The model under review builds one solid part; all positions refer to its coordinate system, in mm. A direction names the side the tool comes from. Round coordinates to 2 decimals unless told otherwise and drop trailing zeros. Order: outer loops, then holes, each group sorted by start corner. A loop starts at its lowest first (then second) coordinate and runs counter-clockwise, first axis right, second up. Notation, with made-up numbers: (-39.5, -10.5) - (9.5, -10.5) arc R16 ccw to (9.5, -4.5) - close; hole circle Ø5 at (87, 48.25). An arc over 180 degrees is marked (long way). One line per question, with ' | ' between items. Start each with the question number.
Item 1: Add section B-B on x = -27.5. State the section outline as (y, z) points.
Item 2: Insertion check: pin 1 Ø3.5 at (y, z) = (-35.5, -5) entering from -X; pin 2 Ø2.5 at (y, z) = (-34.5, -23) entering from +X; pin 3 Ø3.5 at (y, z) = (-35, -6.5) entering from +X. Each pin has a flat end and moves straight along its axis. Give the tip position at first contact, or say it passes through.
Item 3: Add section A-A on z = -4.5. State the section outline as (x, y) points.
Item 4: Draft analysis for pull direction Y (two halves, no side actions). For faces 4 (the face through (-30, 35, -1.58)), 5 (the face through (-16, 36.25, -12)), 6 (the face through (80, 0, -4)), state which applies: +Y half, -Y half, draft (parallel to the pull), parting line (faces both ways), or undercut.
Item 5: For L1, parallel to Y at x = -38, z = -30.5; L2, parallel to X at y = -28, z = -2; L3, parallel to X at y = -30, z = -9.5, list the stretches that pass through material, from the lowest coordinate up. Write a range as [from, to].
Item 6: Tool access review of faces 1 (the face through (-66, -35, -1.093)), 2 (the face through (-80, 0, -17)), 3 (the face through (-47.3, 35, -17)): name each direction out of +Z, -Z, +X, -X, +Y, -Y from which nothing blocks a thin tool from reaching the whole face with its end or side.
Item 7: Add section C-C on y = 6.5. State the section outline as (x, z) points, and give its area (3 significant figures).
Item 8: Add section D-D on x = -9. State the section outline as (y, z) points, and give its area (3 significant figures).
from build123d import *

# Parameters (mm, degrees)
ESQUISSE1_W                  = 160
ESQUISSE1_H                  = 66.5
BOSS_EXTRU_1_DEPTH           = 3
ESQUISSE3_W                  = 3
ESQUISSE3_H                  = 70.75
BOSS_EXTRU_2_DEPTH           = 33
ESQUISSE5_W                  = 166
ESQUISSE5_H                  = 33
ESQUISSE5_W_2                = 11.569169734
ESQUISSE5_H_2                = 9.894756015
BOSS_EXTRU_3_DEPTH           = 3
ENL_V_MAT_EXTRU_1_DEPTH      = 500
ENL_V_MAT_EXTRU_1_DEPTH_BACK = 13
ESQUISSE6_W                  = 33
ESQUISSE6_H                  = 1.25
CONG_2_R                     = 4
ESQUISSE7_W                  = 98.078954594
ESQUISSE7_H                  = 17.67
ENL_V_MAT_EXTRU_2_DEPTH      = 103
ESQUISSE8_R                  = 3.75
ENL_V_MAT_EXTRU_3_DEPTH      = 60
ESQUISSE9_W                  = 103.919717687
ESQUISSE9_H                  = 4.5
ENL_V_MAT_EXTRU_4_DEPTH      = 90
ESQUISSE11_W                 = 11.569169734
ESQUISSE11_H                 = 9.894756015
BOSS_EXTRU_4_DEPTH           = 3
D_PLACER_START               = -33.9
D_PLACER_LA_FACE2_DEPTH      = 3.9
ESQUISSE13_W                 = 16.502074088
ESQUISSE13_H                 = 4.3431
ENL_V_MAT_EXTRU_5_DEPTH      = 10
ESQUISSE15_W                 = 9.760998185
ESQUISSE15_H                 = 7
ENL_V_MAT_EXTRU_6_DEPTH      = 10


# Read off the part's stored shape, not the designer's step: Déplacer la face2
with BuildPart() as part:
    # Esquisse1 → Boss.-Extru.1 (new body)
    with BuildSketch(Plane.XY):
        Rectangle(ESQUISSE1_W, ESQUISSE1_H)
    extrude(amount=BOSS_EXTRU_1_DEPTH)

    # Esquisse3 → Boss.-Extru.2 (add)
    with BuildSketch(Plane.XY.offset(3)):
        with Locations((-81.5, -2.125)):
            Rectangle(ESQUISSE3_W, ESQUISSE3_H)
    boss_extru_2 = extrude(amount=-BOSS_EXTRU_2_DEPTH)

    # Symétrie1: Boss.-Extru.2 across plane
    add(boss_extru_2.mirror(Plane(origin=(0, 0, 0), x_dir=(0, 0, 1), z_dir=(1, 0, 0))))

    # Esquisse5 → Boss.-Extru.3 (add)
    with BuildSketch(Plane(origin=(0, 33.25, 0), x_dir=(1, 0, 0), z_dir=(0, 1, 0))):
        with Locations((0, 13.5)):
            Rectangle(ESQUISSE5_W, ESQUISSE5_H)
        with Locations((-29.852297111, 6.527378008)):
            Rectangle(ESQUISSE5_W_2, ESQUISSE5_H_2, mode=Mode.SUBTRACT)
    boss_extru_3 = extrude(amount=BOSS_EXTRU_3_DEPTH)

    # Symétrie2: Boss.-Extru.3 across plane
    add(boss_extru_3.mirror(Plane(origin=(0, 0, 0), x_dir=(0, 0, 1), z_dir=(0, -1, 0))))

    # Esquisse6 → Enlèv. mat.-Extru.1 (cut, two sides: drawn at the far end of the back side and taken through both)
    with BuildSketch(Plane.ZY.offset(-80).offset(-ENL_V_MAT_EXTRU_1_DEPTH_BACK)):
        with Locations((-13.5, -36.875)):
            Rectangle(ESQUISSE6_W, ESQUISSE6_H)
    extrude(amount=ENL_V_MAT_EXTRU_1_DEPTH + ENL_V_MAT_EXTRU_1_DEPTH_BACK, mode=Mode.SUBTRACT)

    # Congé2
    cong_2_edges = [part.edges().sort_by_distance(p)[0] for p in [
        (-83, -36.25, -13.5),
        (83, -36.25, -13.5),
        (-83, 36.25, -13.5),
        (83, 36.25, -13.5),
    ]]
    fillet(cong_2_edges, radius=CONG_2_R)

    # Esquisse7 → Enlèv. mat.-Extru.2 (cut)
    with BuildSketch(Plane(origin=(0, 36.25, 0), x_dir=(1, 0, 0), z_dir=(0, 1, 0))):
        with Locations((35.039477297, 21.165)):
            Rectangle(ESQUISSE7_W, ESQUISSE7_H)
    extrude(amount=-ENL_V_MAT_EXTRU_2_DEPTH, mode=Mode.SUBTRACT)

    # Esquisse8 → Enlèv. mat.-Extru.3 (cut)
    with BuildSketch(Plane.ZY.offset(83)):
        with Locations(Location((-23.114912873, -22.364838355, 0), (0, 0, 270))):
            Circle(ESQUISSE8_R)
        with Locations(Location((-23.117764577, 1.001660884, 0), (0, 0, 270))):
            Circle(ESQUISSE8_R)
    extrude(amount=-ENL_V_MAT_EXTRU_3_DEPTH, mode=Mode.SUBTRACT)

    # Esquisse9 → Enlèv. mat.-Extru.4 (cut)
    with BuildSketch(Plane(origin=(0, 36.25, 0), x_dir=(1, 0, 0), z_dir=(0, 1, 0))):
        with Locations((37.959858844, 10.08)):
            Rectangle(ESQUISSE9_W, ESQUISSE9_H)
    extrude(amount=-ENL_V_MAT_EXTRU_4_DEPTH, mode=Mode.SUBTRACT)

    # Esquisse11 → Boss.-Extru.4 (add)
    with BuildSketch(Plane.XZ.offset(36.25)):
        with Locations((-29.852297111, -6.527378008)):
            Rectangle(ESQUISSE11_W, ESQUISSE11_H)
    extrude(amount=-BOSS_EXTRU_4_DEPTH)

    # Déplacer la face2 outline → Déplacer la face2 (add)
    with BuildSketch(Plane.XY.offset(D_PLACER_START)):
        with BuildLine():
            ThreePointArc((-79, 36.25), (-81.828427125, 35.078427125), (-83, 32.25))
            Line((-83, 32.25), (-83, -32.25))
            ThreePointArc((-83, -32.25), (-81.828427125, -35.078427125), (-79, -36.25))
            Line((-79, -36.25), (-14, -36.25))
            Line((-14, -36.25), (-14, -33.25))
            Line((-14, -33.25), (-80, -33.25))
            Line((-80, -33.25), (-80, 33.25))
            Line((-80, 33.25), (-14, 33.25))
            Line((-14, 33.25), (-14, 36.25))
            Line((-14, 36.25), (-79, 36.25))
        make_face()
    extrude(amount=D_PLACER_LA_FACE2_DEPTH)

    # Esquisse13 → Enlèv. mat.-Extru.5 (cut)
    with BuildSketch(Plane(origin=(0, 36.25, 0), x_dir=(1, 0, 0), z_dir=(0, 1, 0))):
        with Locations((-55.551088515, 16.608317679)):
            Rectangle(ESQUISSE13_W, ESQUISSE13_H)
    extrude(amount=-ENL_V_MAT_EXTRU_5_DEPTH, mode=Mode.SUBTRACT)

    # Esquisse15 → Enlèv. mat.-Extru.6 (cut)
    with BuildSketch(Plane.XZ.offset(36.25)):
        with Locations((-66.304513779, -4.593344901)):
            Rectangle(ESQUISSE15_W, ESQUISSE15_H)
    extrude(amount=-ENL_V_MAT_EXTRU_6_DEPTH, mode=Mode.SUBTRACT)


solid = part.part
Determined:
1) outline: (-36.25, -33.9) - (-33.25, -33.9) - (-33.25, 0) - (33.25, 0) - (33.25, -1.58) - (36.25, -1.58) - (36.25, 3) - (-36.25, 3) - close; (33.25, -33.9) - (36.25, -33.9) - (36.25, -11.47) - (33.25, -11.47) - close
2) pin 1: x = -82.71 | pin 2: x = -14 | pin 3: x = 82.87
3) outline: (-83, -32.25) arc R4 ccw to (-79, -36.25) - (-71.19, -36.25) - (-71.19, -33.25) - (-80, -33.25) - (-80, 33.25) - (-35.64, 33.25) - (-35.64, 36.25) - (-79, 36.25) arc R4 ccw to (-83, 32.25) - close; (-61.42, -36.25) - (79, -36.25) arc R4 ccw to (83, -32.25) - (83, 32.25) arc R4 ccw to (79, 36.25) - (-24.07, 36.25) - (-24.07, 33.25) - (80, 33.25) - (80, -33.25) - (-61.42, -33.25) - close
4) face 4: draft | face 5: +Y half | face 6: undercut
5) L1: [-36.25, -33.25], [33.25, 36.25] | L2: [-83, -80], [80, 83] | L3: [-83, -80]
6) face 1: -Y | face 2: -Z | face 3: +Y
7) outline: (-83, -33.9) - (-80, -33.9) - (-80, 0) - (80, 0) - (80, -7.83) - (83, -7.83) - (83, 3) - (-83, 3) - close | area: 623 mm2
8) outline: (-36.25, -7.83) - (-33.25, -7.83) - (-33.25, 0) - (33.25, 0) - (33.25, -7.83) - (36.25, -7.83) - (36.25, 3) - (-36.25, 3) - close | area: 264 mm2
